The model under review builds one solid part; all positions refer to its coordinate system, in mm. Face numbers are marked on the shaded views. A direction names the side the tool comes from. Round coordinates to 2 decimals unless told otherwise and drop trailing zeros. Loops run counter-clockwise (first coordinate to the right, second up) from the corner with the lowest first, then second, coordinate; pieces in that order, holes last. Notation, with made-up numbers: (41, 67.25) -> (56, 67.25) arc R13 ccw to (56, 92.25) -> close; hole circle Ø3 at (-13.75, 71). An arc over 180 degrees is marked (long way). Write each question's results on one line, items separated by ' | '. Start each with the question number.
Item 1: For L1, parallel to X at y = -1.5, z = -7.25; L2, parallel to X at y = -0.82, z = -5.25; L3, parallel to Z at x = -25, y = 18.25, list the stretches that pass through material, from the lowest coordinate up. Write a range as from..to.
Item 2: We need section A-A (x = 5.5). Give the boundary of the cut face in (y, z).
Item 3: Tool access review of the marked faces 1, 2 and 3: name each direction out of +Z, -Z, +X, -X, +Y, -Y from which nothing blocks a thin tool from reaching the whole face with its end or side.
Item 4: We need section C-C (z = 2). Give the boundary of the cut face in (x, y).
Item 5: Clearance check with flat-ended pins moving along their axes: pin 1 Ø4 at (x, y) = (-16, 10.5) entering from +Z; pin 2 Ø10.5 at (x, y) = (22.5, 13.5) entering from -Z; pin 3 Ø1.5 at (x, y) = (12, 0) entering from -Z. State where each tip first meets the part, or that it passes through.
Item 6: We need section B-B (y = -0.82). Give the boundary of the cut face in (x, z), and give its area (3 significant figures).
Item 7: We need section D-D (x = -11.75). Give the boundary of the cut face in (y, z).
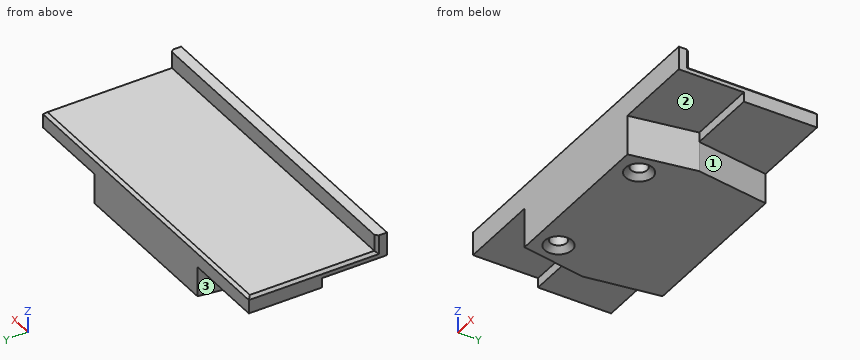
from build123d import *

# Parameters (mm, degrees)
SKETCH025_W          = 25.23103
SKETCH025_H          = 60
PAD004_DEPTH         = 3
PAD005_DEPTH         = 5.5
SKETCH027_R          = 1.5
POCKET005_DEPTH      = 7.25
SKETCH028_W          = 2
SKETCH028_H          = 60
PAD006_DEPTH         = 3
POCKET006_DEPTH      = 1.75
CHAMFER003_SIZE      = 0.5
CHAMFER004_SIZE      = 1
BODY_ROLL_ANGLE      = -180
BODY_PLACEMENT_ANGLE = -90


with BuildPart() as part:
    # Sketch025 → Pad004 (new body)
    with BuildSketch(Plane.XY):
        with Locations((-10.615515, 0)):
            Rectangle(SKETCH025_W, SKETCH025_H)
    extrude(amount=PAD004_DEPTH)

    # Sketch026 (on Face6 of Pad004) → Pad005 (join)
    with BuildSketch(Plane.XY.offset(3)):
        Polygon((-23.23103, 15), (-9.88, 17), (2, 15), (2, -15), (-9.88, -17), (-23.23103, -15), align=None)
    extrude(amount=PAD005_DEPTH)

    # Sketch027 (on Face12 of Pad005) → Pocket005 (cut)
    with BuildSketch(Plane.XY.offset(8.5)):
        with Locations((-2.18, 11.75)):
            Circle(SKETCH027_R)
        with Locations((-2.18, -11.75)):
            Circle(SKETCH027_R)
    extrude(amount=-POCKET005_DEPTH, mode=Mode.SUBTRACT)

    # Sketch028 (on Face4 of Pocket005) → Pad006 (join)
    with BuildSketch(Plane(origin=(0, 0, 0), x_dir=(1, 0, 0), z_dir=(0, 0, -1))):
        with Locations((1, 0)):
            Rectangle(SKETCH028_W, SKETCH028_H)
    extrude(amount=PAD006_DEPTH)

    # Sketch029 (on Face9 of Pad006) → Pocket006 (cut)
    with BuildSketch(Plane.XY.offset(3)):
        Polygon((2, 30), (-9.88, 30), (-9.88, 17), (2, 15), align=None)
        Polygon((2, -30), (2, -15), (-9.88, -17), (-9.88, -30), align=None)
    extrude(amount=-POCKET006_DEPTH, mode=Mode.SUBTRACT)

    # Chamfer003
    chamfer003_edges = [part.edges().sort_by_distance(p)[0] for p in [
        (0, 30, -1.5),
        (0, -30, -1.5),
        (-11.615515, 30, 0),
        (-23.23103, 0, 0),
        (-11.615515, -30, 0),
    ]]
    chamfer(chamfer003_edges, length=CHAMFER003_SIZE)

    # Chamfer004
    chamfer004_edges = [part.edges().sort_by_distance(p)[0] for p in [
        (-3.68, -11.75, 8.5),
        (-3.68, 11.75, 8.5),
    ]]
    chamfer(chamfer004_edges, length=CHAMFER004_SIZE)


with BuildPart() as part_1:
    # Body roll: moved
    add(part.part.rotate(Axis((0, 0, 0), (1, 0, 0)), BODY_ROLL_ANGLE))


with BuildPart() as part_2:
    # Body placement: moved
    add(part_1.part.moved(Location((0, -3, 0))).rotate(Axis((0, -3, 0), (0, 0, 1)), BODY_PLACEMENT_ANGLE))


solid = part_2.part
Here are the results:
1) L1: x = -15.59..-13.09, -10.41..10.41, 13.09..15.59 | L2: x = -15.7..-13.25, -10.25..10.25, 13.25..15.7 | L3: z = -3..0
2) outline: (-5, -8.5) -> (20.23, -8.5) -> (20.23, -0.5) -> (19.73, 0) -> (-3, 0) -> (-3, 3) -> (-5, 3) -> close
3) face 1: -Z, +X, +Y | face 2: -Z, +X, -Y | face 3: -Z, -X, +Y
4) outline: (-30, -5) -> (30, -5) -> (30, -3.5) -> (29.5, -3) -> (-29.5, -3) -> (-30, -3.5) -> close
5) pin 1: stops at z = 0 | pin 2: stops at z = -3 | pin 3: stops at z = -7.61
6) outline: (-30, -1.25) -> (-15.7, -1.25) -> (-15.7, -8.5) -> (-14.25, -8.5) -> (-13.25, -7.5) -> (-13.25, -1.25) -> (-10.25, -1.25) -> (-10.25, -7.5) -> (-9.25, -8.5) -> (9.25, -8.5) -> (10.25, -7.5) -> (10.25, -1.25) -> (13.25, -1.25) -> (13.25, -7.5) -> (14.25, -8.5) -> (15.7, -8.5) -> (15.7, -1.25) -> (30, -1.25) -> (30, -0.5) -> (29.5, 0) -> (-29.5, 0) -> (-30, -0.5) -> close | area: 257 mm2
7) outline: (-5, -8.5) -> (-3.32, -8.5) -> (-2.32, -7.5) -> (-2.32, -1.25) -> (0.68, -1.25) -> (0.68, -7.5) -> (1.68, -8.5) -> (20.23, -8.5) -> (20.23, -0.5) -> (19.73, 0) -> (-3, 0) -> (-3, 3) -> (-5, 3) -> close
